Answer from the drawing. Dimensions are ordinates in mm from the lowest x, y and z of the part. A direction names the side the tool comes from. Coordinates: 2 decimals unless noted, no trailing zeros. Write each loop counter-clockwise with the first axis right and the second up, starting at its lowest first coordinate (ties: lowest second). Pieces come first, ordered by that corner, then holes.
(1) Straight lines are drawn through the part: line 1 (Y direction, x = 88, z = 4.75) (1 decimal); line 2 (Y direction, x = 95, z = 12.25) (1 decimal); line 3 (Z direction, x = 7, y = 8). For each, find the intervals that lie inside material, in ascending order.
(2) Given P1, Ø4, axis at x = 44, z = 10, coming from the +Y side; P2, Ø1.5, axis at x = 83, z = 16.5, coming from the +Y side, each flat-ended and moving along its own axis, determine where each tip first touches the part or whether it passes through.
(3) The part is cut by section A-A on x = 67.5. Determine the outline of the cut face in (y, z) (1 decimal).
(4) Which of the six approach directions +Z, -Z, +X, -X, +Y, -Y give full straight-line access (tool end or side, diameter ignored) to the marked faces 1, 2 and 3?
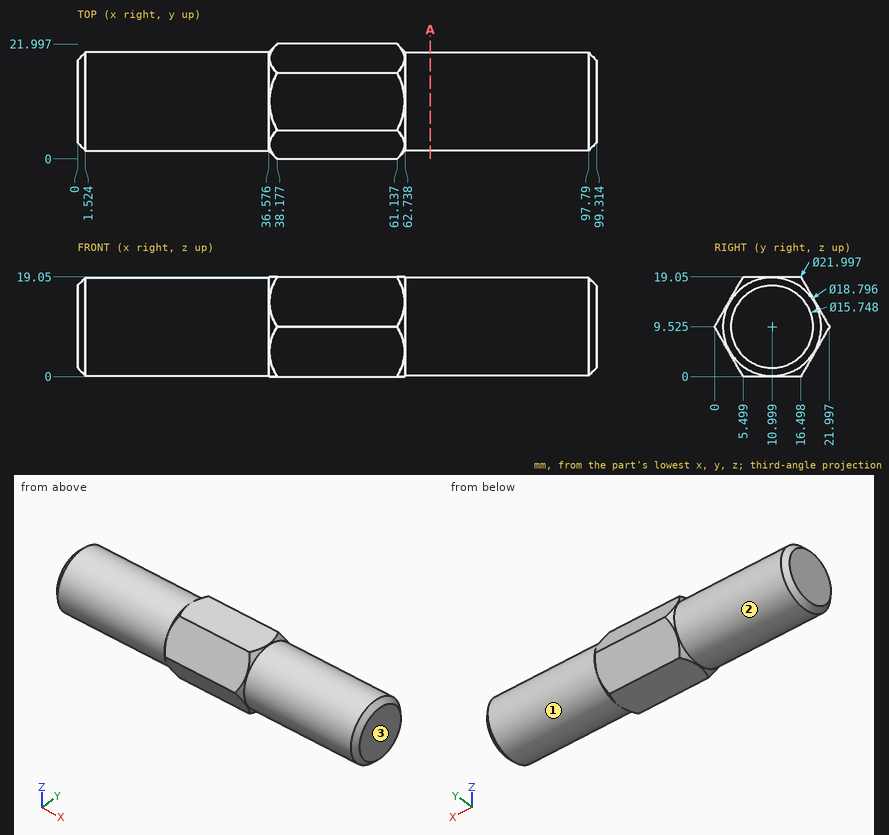
Model answer:
1. line 1: y = 2.9 to 19.1
1. line 2: y = 2 to 20
1. line 3: z = 0.62 to 18.43
2. P1: stops at y = 22
2. P2: stops at y = 18.04
3. outline: circle Ø18.8 at (11, 9.5)
4. face 1: +X
4. face 2: -X
4. face 3: +Z, -Z, +X, +Y, -Y
